Can you work these out from the model? Positions are in its coordinate system, mm. A direction names the side the tool comes from. Give positions to 0.01 mm unless a question says otherwise; leave off trailing zeros. Write each loop counter-clockwise with the first axis right and the second up, starting at its lowest first coordinate (ties: lowest second). Pieces come first, ordered by that corner, then holes. Notation, with made-up numbers: (11, -22) - (51, -22) arc R4 cw to (51, -16) - close; hole circle Ø9 at (-18.75, 49). An arc over 180 degrees is marked (long way). Use a Markdown table: item, result. Add a question column.
```python
from build123d import *

# Parameters (mm, degrees)
F1_W     = 207.582682
F1_H     = 126.610666
F2_W     = 123.456738
F2_H     = 75.831934
F5_DEPTH = 60.452
F6_W     = 207.582682
F6_H     = 126.610666
F7_DEPTH = 16.764
F8_DEPTH = 8.636


with BuildPart() as f3:
    # F1 (on Top) → F3 section 0
    with BuildSketch(Plane.XY):
        Rectangle(F1_W, F1_H)
    # F2 (on offset) → F3 section 1
    with BuildSketch(Plane.XY.offset(86.36)):
        Rectangle(F2_W, F2_H)
    loft()

    # F4 (on Front) → F5 (join, symmetric)
    with BuildSketch(Plane.XZ):
        with BuildLine():
            Line((-48.884847, 20.875009), (48.884847, 20.875009))
            ThreePointArc((48.884847, 20.875009), (0, 69.759856), (-48.884847, 20.875009))
        make_face()
    extrude(amount=F5_DEPTH, both=True)

    # F6 (on face) → F7 (join)
    with BuildSketch(Plane(origin=(0, 0, 0), x_dir=(1, 0, 0), z_dir=(0, 0, -1))):
        Rectangle(F6_W, F6_H)
    extrude(amount=F7_DEPTH)

    # F4 (on Front) → F8 (join, symmetric)
    with BuildSketch(Plane.XZ):
        Polygon((22.331208, 186.080039), (-26.018247, 84.848367), (-29.040085, 81.322886), (28.374884, 81.322886), (74.206144, 186.080039), align=None)
    extrude(amount=F8_DEPTH, both=True)


solid = f3.part
```
Q1. Suppose I cut it at B-B (z = 116). Please give me the cut outline in (x, y), and give its area (3 significant figures).
Q2. I'm going to push flat-ended pins straight in: P1, Ø1.5, axis at x = -18, z = 101, coming from the +Y side; P2, Ø6, axis at y = 29.5, z = 51, coming from the +X side; P3, Ø5, axis at x = 40, y = 28.5, coming from the +Z side. Where does each tip first touch, or does it pass through?
Q3. Suppose I cut it at A-A (z = 171). Please give me the cut outline in (x, y).
Q4. If I drill on probe 1 along Y at (x, z) = (51.5, 140); probe 2 along Y at (x, z) = (-30, 34.5); probe 3 along Z at (x, y) = (38, -33), over which ranges is the centre line in solid material (lowest first)? Write a range as [from, to].
Q5. On a 3-axis mill with a long thin cutter (end or side, diameter ignored), from which of +Z, -Z, +X, -X, +Y, -Y can I reach the whole of each face in a straight line? I mean faces 1 (the flat face through (-1, -60.452, 40)), 2 (the cylindrical face through (1.07, 53.46, 69.75)), 3 (the flat face through (-1, 60.452, 40)), 4 (the flat face through (52.087, -0.121, 135.522)). Say none if no direction works.
Derived:
| question | item | result |
|---|---|---|
| 1 | outline | (-11.14, -8.64) - (43.55, -8.64) - (43.55, 8.64) - (-11.14, 8.64) - close |
| 1 | area | 945 mm² |
| 2 | P1 | y = 8.64 |
| 2 | P2 | x = 80.41 |
| 2 | P3 | z = 86.36 |
| 3 | outline | (15.13, -8.64) - (67.61, -8.64) - (67.61, 8.64) - (15.13, 8.64) - close |
| 4 | probe 1 | [-8.64, 8.64] |
| 4 | probe 2 | [-60.45, 60.45] |
| 4 | probe 3 | [-16.76, 86.36] |
| 5 | face 1 | +Z, +X, -X, -Y |
| 5 | face 2 | +Z, +Y |
| 5 | face 3 | +Z, +X, -X, +Y |
| 5 | face 4 | +X, +Y, -Y |
